Work out the finished part from the listing and answer in its coordinate system (mm). Face numbers are marked on the shaded views. A direction names the side the tool comes from. Give positions to 0.01 mm unless a question says otherwise; leave off trailing zeros. Loops run counter-clockwise (first coordinate to the right, second up) from the corner with the lowest first, then second, coordinate; pieces in that order, holes last. Notation, with made-up numbers: M -17,4 L 4,4 A26 cw 4,42 Z; hole C 16.5,48.5 d1. An arc over 180 degrees is marked long. Write item = value, one per line. Start each with the question number.
1. Section D-D on y = 3 is taken. Give the number of separate pieces and of enclosed holes in the cut face, plus the area to 3 significant figures.
2. Section B-B on x = 10.5 is taken. Determine the outline of the cut face in (y, z), plus the area to 3 significant figures.
3. For the marked faces 1, 2 and 3, determine the directions among +Z, -Z, +X, -X, +Y, -Y from which every point of the face is accessible in a straight line to the end or side of a thin tool.
4. Section A-A on z = -38 is taken. Determine the outline of the cut face in (x, y), plus the area to 3 significant figures.
5. The mould has two halves that part along X. Classify the marked faces 4, 5 and 6: released by +X, released by -X, zero draft, split by the parting line, or undercut.
6. Consider L1, parallel to X at y = 6.5, z = -53.5; L2, parallel to Z at x = 30, y = 9; L3, parallel to X at y = 3.5, z = 49.3. Determine where each line is inside the solid, lowest interval first. Write a range as [from, to].
7. Flat-ended cylindrical pins translate along their axes: pin 1 Ø9 at (x, z) = (-27.12, 60.5) entering from -Y; pin 2 Ø2 at (x, y) = (10.5, 38) entering from -Z; pin 3 Ø10 at (y, z) = (32, -35) entering from -X. Find the tip coordinate at first contact, or state that the pin passes through.
8. Section C-C on y = 30 is taken. Determine the outline of the cut face in (x, z), plus the area to 3 significant figures.
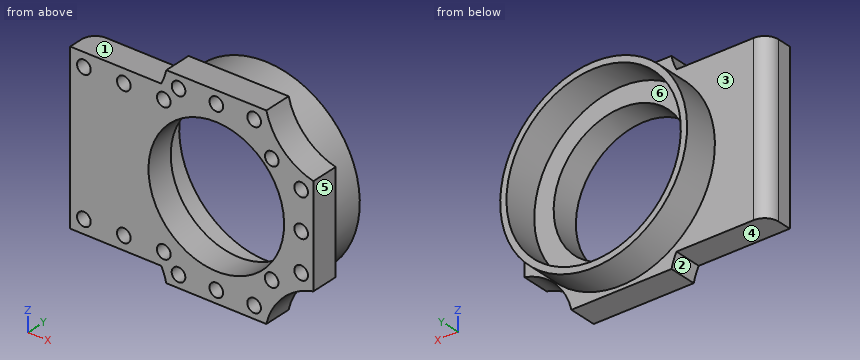
```python
from build123d import *

# Parameters (mm, degrees)
SALIENTE_EXTRUIR4_DEPTH = 20
REDONDEO1_R             = 10
CROQUIS4_3_R            = 4.9
CORTAR_EXTRUIR3_DEPTH   = 10
CROQUIS7_R              = 67.17
CROQUIS7_R_2            = 62.67
SALIENTE_EXTRUIR7_DEPTH = 25
CROQUIS8_R              = 48.75
CORTAR_EXTRUIR4_DEPTH   = 129.538087741


with BuildPart() as part:
    # Croquis2 → Saliente-Extruir4 (new body)
    with BuildSketch(Plane(origin=(0, 0, 0), x_dir=(1, 0, 0), z_dir=(0, 1, 0))):
        with BuildLine():
            Line((-105, 59.8), (-105, -59.1))
            Line((-105, -59.1), (-39.564866762, -59.1))
            ThreePointArc((-39.564866762, -59.1), (-37.4362836, -64.089147092), (-35.920673767, -69.297350411))
            Line((-35.920673767, -69.297350411), (36.010468241, -69.60956711))
            ThreePointArc((36.010468241, -69.60956711), (48.107993991, -47.969702582), (69.8, -35.965922287))
            Line((69.8, -35.965922287), (69.8, 35.965922287))
            ThreePointArc((69.8, 35.965922287), (48.03877349, 48.03877349), (35.965922287, 69.8))
            Line((35.965922287, 69.8), (-35.965922287, 69.8))
            ThreePointArc((-35.965922287, 69.8), (-37.470458506, 64.693854165), (-39.564866762, 59.8))
            Line((-39.564866762, 59.8), (-105, 59.8))
        make_face()
    extrude(amount=SALIENTE_EXTRUIR4_DEPTH)

    # Redondeo1
    redondeo1_edges = [part.edges().sort_by_distance(p)[0] for p in [
        (-105, 20, -0.35),
    ]]
    fillet(redondeo1_edges, radius=REDONDEO1_R)

    # Croquis4_3 → Cortar-Extruir3 (cut)
    with BuildSketch(Plane.XZ):
        with Locations(Location((-95.2, 49.3, 0), (0, 0, 270))):
            Circle(CROQUIS4_3_R)
        with Locations(Location((-66.482433381, 49.3, 0), (0, 0, 270))):
            Circle(CROQUIS4_3_R)
        with Locations(Location((-37.764866762, 49.3, 0), (0, 0, 270))):
            Circle(CROQUIS4_3_R)
        with Locations(Location((-27.120673767, 60.497350411, 0), (0, 0, 270))):
            Circle(CROQUIS4_3_R)
        with Locations(Location((0.044897237, 60.497350411, 0), (0, 0, 270))):
            Circle(CROQUIS4_3_R)
        with Locations(Location((27.210468241, 60.497350411, 0), (0, 0, 270))):
            Circle(CROQUIS4_3_R)
        with Locations(Location((61, 27.165922287, 0), (0, 0, 270))):
            Circle(CROQUIS4_3_R)
        with Locations(Location((39.878985668, 39.547302783, 0), (0, 0, 270))):
            Circle(CROQUIS4_3_R)
        with Locations(Location((61, 0, 0), (0, 0, 270))):
            Circle(CROQUIS4_3_R)
        with Locations(Location((61, -27.165922287, 0), (0, 0, 270))):
            Circle(CROQUIS4_3_R)
        with Locations(Location((27.165922287, -61, 0), (0, 0, 270))):
            Circle(CROQUIS4_3_R)
        with Locations(Location((39.753243225, -39.753243225, 0), (0, 0, 270))):
            Circle(CROQUIS4_3_R)
        with Locations(Location((0, -61, 0), (0, 0, 270))):
            Circle(CROQUIS4_3_R)
        with Locations(Location((-27.165922287, -61, 0), (0, 0, 270))):
            Circle(CROQUIS4_3_R)
        with Locations(Location((-37.764866762, -50, 0), (0, 0, 270))):
            Circle(CROQUIS4_3_R)
        with Locations(Location((-66.482433381, -50, 0), (0, 0, 270))):
            Circle(CROQUIS4_3_R)
        with Locations(Location((-95.2, -50, 0), (0, 0, 270))):
            Circle(CROQUIS4_3_R)
    extrude(amount=-CORTAR_EXTRUIR3_DEPTH, mode=Mode.SUBTRACT)

    # Croquis7 → Saliente-Extruir7 (add)
    with BuildSketch(Plane(origin=(0, 20, 0), x_dir=(1, 0, 0), z_dir=(0, 1, 0))):
        with Locations(Location((0, 0, 0), (0, 0, 270))):
            Circle(CROQUIS7_R)
        with Locations(Location((0, 0, 0), (0, 0, 270))):
            Circle(CROQUIS7_R_2, mode=Mode.SUBTRACT)
    extrude(amount=SALIENTE_EXTRUIR7_DEPTH)

    # Croquis8 → Cortar-Extruir4 (cut, through all)
    with BuildSketch(Plane(origin=(0, 20, 0), x_dir=(1, 0, 0), z_dir=(0, 1, 0))):
        with Locations(Location((0, 0, 0), (0, 0, 270))):
            Circle(CROQUIS8_R)
    extrude(amount=-CORTAR_EXTRUIR4_DEPTH, mode=Mode.SUBTRACT)


solid = part.part
```
Verdict:
q1.separate_pieces = 1
q1.enclosed_holes = 18
q1.area = 12,600 mm2
q2.outline = M 0,-69.8 L 20,-69.8 L 20,-66.34 L 45,-66.34 L 45,-61.78 L 20,-61.78 L 20,-47.61 L 0,-47.61 Z; M 0,47.61 L 20,47.61 L 20,61.78 L 45,61.78 L 45,66.34 L 20,66.34 L 20,69.5 L 0,69.5 Z
q2.area = 1,110 mm2
q3.face_1 = +Z, -X, +Y, -Y
q3.face_2 = -Z, -X, +Y, -Y
q3.face_3 = +Y
q4.outline = M -105,0 L -30.54,0 L -30.54,20 L -49.84,20 L -49.84,45 L -55.39,45 L -55.39,20 L -95,20 A10 ccw -105,10 Z; M 30.54,0 L 35.18,0 L 35.18,10 L 44.33,10 L 44.33,0 L 63.3,0 L 63.3,20 L 55.39,20 L 55.39,45 L 49.84,45 L 49.84,20 L 30.54,20 Z
q4.area = 2,310 mm2
q5.face_4 = zero draft
q5.face_5 = released by +X
q5.face_6 = undercut
q6.L1 = [-105, -98.63], [-91.77, -69.91], [-63.05, -41.19], [-34.34, 43.38]
q6.L2 = [-69.8, -65], [-57, -38.43], [38.43, 56.47], [64.53, 69.58]
q6.L3 = [-105, -100.1], [-90.3, -71.38], [-61.58, -42.66], [-32.86, 46.83]
q7.pin_1 = 10
q7.pin_2 = -66.49
q7.pin_3 = -60.1
q8.outline = C 0,0 d134.34; hole C 0,0 d125.34
q8.area = 1,840 mm2
